from build123d import *

# Parameters (mm, degrees)
EXTRUDE_1_DEPTH           = 25
SKETCH_4_R                = 2.5
CUT_EXTRUDE_1_DEPTH       = 50
HOLE_WIZARD_2_D           = 4.5
HOLE_WIZARD_2_CBORE_D     = 8
HOLE_WIZARD_2_CBORE_DEPTH = 4.6


with BuildPart() as part:
    # 草图1 → 凸台-拉伸1 (new, symmetric)
    with BuildSketch(Plane.XY):
        Polygon((-28.5, 2), (-28.5, 14), (-38.5, 14), (-38.5, 0), (38.5, 0), (38.5, 14), (28.5, 14), (28.5, 2), align=None)
    extrude(amount=EXTRUDE_1_DEPTH, both=True)

    # 草图4 → 切除-拉伸1 (cut, symmetric)
    with BuildSketch(Plane(origin=(0, 0, 0), x_dir=(0, 0, -1), z_dir=(1, 0, 0))):
        with Locations(Location((18, 9, 0), (0, 0, 90))):
            Circle(SKETCH_4_R)
        with Locations(Location((-13, 9, 0), (0, 0, 90))):
            Circle(SKETCH_4_R)
    extrude(amount=CUT_EXTRUDE_1_DEPTH, both=True, mode=Mode.SUBTRACT)

    # 打孔尺寸根据内六角圆柱头螺钉的类型2 (through all)
    with Locations(Plane(origin=(0, 14, 0), x_dir=(-1, 0, 0), z_dir=(0, 1, 0))):
        with Locations((33.5, -11), (33.5, 20)):
            hole_wizard_2 = CounterBoreHole(HOLE_WIZARD_2_D / 2, HOLE_WIZARD_2_CBORE_D / 2, HOLE_WIZARD_2_CBORE_DEPTH)

    # 镜向2: 打孔尺寸根据内六角圆柱头螺钉的类型2 across plane
    add(hole_wizard_2.mirror(Plane(origin=(0, 0, 0), x_dir=(0, 0, 1), z_dir=(1, 0, 0))), mode=Mode.SUBTRACT)


solid = part.part
Verification items for the finished model (mm, model axes). A direction names the side the tool comes from. Round coordinates to 2 decimals unless told otherwise and drop trailing zeros. Write each loop counter-clockwise with the first axis right and the second up, starting at its lowest first coordinate (ties: lowest second). Pieces come first, ordered by that corner, then holes.
(1) Section check D-D (y = 1). Enter the section's corners in (x, z), plus the area to 3 significant figures.
Returned:
outline: (-38.5, -25) - (38.5, -25) - (38.5, 25) - (-38.5, 25) - close; hole circle Ø4.5 at (-33.5, -11); hole circle Ø4.5 at (-33.5, 20); hole circle Ø4.5 at (33.5, -11); hole circle Ø4.5 at (33.5, 20)
area: 3,790 mm2
(2) Section check A-A (z = 11.5). Enter the section's corners in (x, y), plus the area to 3 significant figures.
Returned:
outline: (-38.5, 0) - (38.5, 0) - (38.5, 7) - (28.5, 7) - (28.5, 2) - (-28.5, 2) - (-28.5, 7) - (-38.5, 7) - close; (-38.5, 11) - (-28.5, 11) - (-28.5, 14) - (-38.5, 14) - close; (28.5, 11) - (38.5, 11) - (38.5, 14) - (28.5, 14) - close
area: 314 mm2
(3) Access from +Z, -Z, +X, -X, +Y, -Y to the whole of each face (thin tool, end or side, straight path). Record for faces 1 (the cylindrical face through (32.29, 4.634, -9.103)), 2 (the flat face through (35, 9.4, 18)).
Returned:
face 1: +Y, -Y
face 2: +Y
(4) Section check B-B (x = -33.5). Enter the section's corners in (y, z).
Returned:
outline: (0, -25) - (14, -25) - (14, -15) - (9.4, -15) - (9.4, -13.25) - (0, -13.25) - close; (0, -8.75) - (9.4, -8.75) - (9.4, -7) - (14, -7) - (14, 16) - (9.4, 16) - (9.4, 17.75) - (0, 17.75) - close; (0, 22.25) - (9.4, 22.25) - (9.4, 24) - (14, 24) - (14, 25) - (0, 25) - close; hole circle Ø5 at (9, -18); hole circle Ø5 at (9, 13)
(5) Section check C-C (y = 8). Give the number of separate pieces and of enclosed holes in the cut face, plus the area to 3 significant figures.
Returned:
separate pieces: 6
enclosed holes: 4
area: 753 mm2
(6) Material ranges on line 1 (Z direction, x = -33.5, y = 11.55); line 2 (Z direction, x = -31, y = 9); line 3 (X direction, y = 4, z = 8.5), recorded low to high.
Returned:
line 1: z = -25 to -15, -7 to 16, 24 to 25
line 2: z = -25 to -20.5, -15.5 to 10.5, 15.5 to 25
line 3: x = -38.5 to -28.5, 28.5 to 38.5
(7) Mould release check, pull along X, two halves, no side actions. Record for faces 3 (the flat face through (-38.5, 7, 0)), 4 (the flat face through (-0.2, 1.8, -25)), 5 (the flat face through (38.5, 7, 0)), 6 (the flat face through (28.5, 8, 0)): pulls with the +X half, pulls with the -X half, needs draft (parallel to the pull), parting line crosses it, or undercut.
Returned:
face 3: pulls with the -X half
face 4: needs draft
face 5: pulls with the +X half
face 6: undercut
(8) Depth check by flat-ended pin: pin 1 Ø4 at (x, z) = (33.5, 20) entering from +Y; pin 2 Ø5 at (x, z) = (33.5, 20) entering from +Y; pin 3 Ø3 at (x, z) = (13.5, 1.5) entering from +Y. Enter the tip coordinate at first touch or a pass-through.
Returned:
pin 1: passes through
pin 2: stops at y = 9.4
pin 3: stops at y = 2
